```python
from build123d import *

# Parameters (mm, degrees)
SKETCH1_W           = 289.69
SKETCH1_H           = 12.7
SKETCH1_R           = 2.49
BOSS_EXTRUDE1_DEPTH = 6.35
FILLET1_R           = 2.54


with BuildPart() as part:
    # Sketch1 → Boss-Extrude1 (new body)
    # profile 1 of 3: a face of its own
    with BuildSketch(Plane(origin=(0, 0, 0), x_dir=(1, 0, 0), z_dir=(0, 1, 0))):
        with Locations((0, -25.4)):
            Rectangle(SKETCH1_W, SKETCH1_H)
        with Locations(Location((138.495, -25.4, 0), (0, 0, 270))):
            Circle(SKETCH1_R, mode=Mode.SUBTRACT)
        with Locations(Location((0, -25.4, 0), (0, 0, 270))):
            Circle(SKETCH1_R, mode=Mode.SUBTRACT)
    # profile 2 of 3: a face of its own
    with BuildSketch(Plane(origin=(0, 0, 0), x_dir=(1, 0, 0), z_dir=(0, 1, 0))):
        Polygon((-144.845, 31.75), (-157.545, 31.75), (-157.545, -31.75), (-144.845, -31.75), (-144.845, -19.05), (-144.845, 19.05), align=None)
        with Locations(Location((-151.195, -25.4, 0), (0, 0, 270))):
            Circle(SKETCH1_R, mode=Mode.SUBTRACT)
        with Locations(Location((-151.195, 25.4, 0), (0, 0, 270))):
            Circle(SKETCH1_R, mode=Mode.SUBTRACT)
    # profile 3 of 3: a face of its own
    with BuildSketch(Plane(origin=(0, 0, 0), x_dir=(1, 0, 0), z_dir=(0, 1, 0))):
        with Locations((0, 25.4)):
            Rectangle(SKETCH1_W, SKETCH1_H)
        with Locations(Location((138.495, 25.4, 0), (0, 0, 270))):
            Circle(SKETCH1_R, mode=Mode.SUBTRACT)
        with Locations(Location((0, 25.4, 0), (0, 0, 270))):
            Circle(SKETCH1_R, mode=Mode.SUBTRACT)
    extrude(amount=BOSS_EXTRUDE1_DEPTH)

    # Fillet1
    fillet1_edges = [part.edges().sort_by_distance(p)[0] for p in [
        (144.845, 3.175, 19.05),
        (144.845, 3.175, 31.75),
        (-157.545, 3.175, 31.75),
        (-157.545, 3.175, -31.75),
        (144.845, 3.175, -31.75),
        (144.845, 3.175, -19.05),
    ]]
    fillet(fillet1_edges, radius=FILLET1_R)


solid = part.part
```
Model file for the job. Use its own axes, mm. A direction names the side the tool comes from. Coordinates: 2 decimals unless noted, no trailing zeros. Write each loop counter-clockwise with the first axis right and the second up, starting at its lowest first coordinate (ties: lowest second). Pieces come first, ordered by that corner, then holes. Notation, with made-up numbers: (13.5, -1) - (35.5, -1) arc R17 cw to (35.5, 14) - close; hole circle Ø1 at (0.5, 88). An arc over 180 degrees is marked (long way). Use a Markdown table: item, result. Add a question column.
Item 1: Band-saw the part on C-C, the plane y = 2.75. Write the cut outline in (x, z) (3 decimals).
Item 2: Two-plate mould, pull along Z, no slides. Class faces 3 (the face through (-8, 3, 31.75)), 4 (the face through (-8, 0, -22)), 5 (the face through (136.064, 3.131, -25.94)): pulls with the +Z half, pulls with the -Z half, needs draft (parallel to the pull), parting line crosses it, or undercut.
Item 3: Band-saw the part on B-B, the plane z = -25.4. Write the cut outline in (x, y) (3 decimals), and give its area (3 significant figures).
Item 4: 3-axis set-ups, long thin cutter, end or side, ignore diameter. For faces 1 (the face through (-144.845, 3, 0)), 2 (the face through (-148.726, 3.131, 25.076)): which of +Z, -Z, +X, -X, +Y, -Y reach the whole face in a straight line?
Item 5: Drill centre lines: line 1 along X through (y, z) = (1.5, 25.4) (3 decimals); line 2 along Z through (x, y) = (54, 3.75); line 3 along X through (y, z) = (0.75, -10) (3 decimals). Where is each one in solid material? Low to high.
Item 6: Band-saw the part on D-D, the plane z = 9.5. Write the cut outline in (x, y) (3 decimals).
Item 7: Band-saw the part on A-A, the plane x = 85. Write the cut outline in (y, z).
A:
| question | item | result |
|---|---|---|
| 1 | outline | (-157.545, -29.21) arc R2.54 ccw to (-155.005, -31.75) - (142.305, -31.75) arc R2.54 ccw to (144.845, -29.21) - (144.845, -21.59) arc R2.54 ccw to (142.305, -19.05) - (-144.845, -19.05) - (-144.845, 19.05) - (142.305, 19.05) arc R2.54 ccw to (144.845, 21.59) - (144.845, 29.21) arc R2.54 ccw to (142.305, 31.75) - (-155.005, 31.75) arc R2.54 ccw to (-157.545, 29.21) - close; hole circle Ø4.98 at (-151.195, -25.4); hole circle Ø4.98 at (-151.195, 25.4); hole circle Ø4.98 at (0, -25.4); hole circle Ø4.98 at (0, 25.4); hole circle Ø4.98 at (138.495, -25.4); hole circle Ø4.98 at (138.495, 25.4) |
| 2 | face 3 | pulls with the +Z half |
| 2 | face 4 | needs draft |
| 2 | face 5 | undercut |
| 3 | outline | (-157.545, 0) - (-153.685, 0) - (-153.685, 6.35) - (-157.545, 6.35) - close; (-148.705, 0) - (-2.49, 0) - (-2.49, 6.35) - (-148.705, 6.35) - close; (2.49, 0) - (136.005, 0) - (136.005, 6.35) - (2.49, 6.35) - close; (140.985, 0) - (144.845, 0) - (144.845, 6.35) - (140.985, 6.35) - close |
| 3 | area | 1,830 mm² |
| 4 | face 1 | +X, +Y, -Y |
| 4 | face 2 | +Y, -Y |
| 5 | line 1 | x = -157.545 to -153.685, -148.705 to -2.49, 2.49 to 136.005, 140.985 to 144.845 |
| 5 | line 2 | z = -31.75 to -19.05, 19.05 to 31.75 |
| 5 | line 3 | x = -157.545 to -144.845 |
| 6 | outline | (-157.545, 0) - (-144.845, 0) - (-144.845, 6.35) - (-157.545, 6.35) - close |
| 7 | outline | (0, -31.75) - (6.35, -31.75) - (6.35, -19.05) - (0, -19.05) - close; (0, 19.05) - (6.35, 19.05) - (6.35, 31.75) - (0, 31.75) - close |
